The listing builds one solid part. Answer for the finished solid, in the listing's coordinates (mm). Give positions to 0.01 mm unless a question says otherwise; leave off trailing zeros. Order: outer loops, then holes, each group sorted by start corner. A loop starts at its lowest first (then second) coordinate and runs counter-clockwise, first axis right, second up. Notation, with made-up numbers: (37, 48) -> (87, 48) arc R28 cw to (87, 82) -> close; hole circle Ø5 at (78, -40). An arc over 180 degrees is marked (long way). One line per question, with ' | ' between items. Start each with the question number.
```python
from build123d import *

# Parameters (mm, degrees)
F0_R     = 0.5
F1_DEPTH = 3.175


# Not quite as in the source:
# - a length typed as a fraction of an inch, garbled in the dataset ("3 / 203.2 mm" for 3/8 in), is restored


with BuildPart() as f1:
    # F0 (on Top) → F1 (new body)
    with BuildSketch(Plane.XY):
        Polygon((-34.3393906951, 49.0726131633), (-37.3393906951, 49.0726131633), (-37.3393906951, 50.5726131633), (-38.8393906951, 50.5726131633), (-38.8393906951, 52.5726131633), (-37.3393906951, 52.5726131633), (-37.3393906951, 61.8976131633), (-41.3393906951, 61.8976131633), (-41.3393906951, 65.0726131633), (-47.3393906951, 65.0726131633), (-47.3393906951, 61.8976131633), (-47.3393906951, -21.1023868367), (-47.3393906951, -24.2773868367), (-41.3393906951, -24.2773868367), (-41.3393906951, -21.1023868367), (-37.3393906951, -21.1023868367), (-37.3393906951, -11.7773868367), (-38.8393906951, -11.7773868367), (-38.8393906951, -9.7773868367), (-37.3393906951, -9.7773868367), (-37.3393906951, -8.2773868367), (-34.3393906951, -8.2773868367), (-34.3393906951, -9.7773868367), (-32.8393906951, -9.7773868367), (-32.8393906951, -11.7773868367), (-34.3393906951, -11.7773868367), (-34.3393906951, -21.1023868367), (-30.3393906951, -21.1023868367), (-30.3393906951, -24.2773868367), (-24.3393906951, -24.2773868367), (-24.3393906951, -21.1023868367), (-24.3393906951, 61.8976131633), (-24.3393906951, 65.0726131633), (-30.3393906951, 65.0726131633), (-30.3393906951, 61.8976131633), (-34.3393906951, 61.8976131633), (-34.3393906951, 52.5726131633), (-32.8393906951, 52.5726131633), (-32.8393906951, 50.5726131633), (-34.3393906951, 50.5726131633), align=None)
        with Locations((-42.4286872149, -2.0273868367)):
            Circle(F0_R, mode=Mode.SUBTRACT)
        with Locations((-42.4286872149, 9.4726131633)):
            Circle(F0_R, mode=Mode.SUBTRACT)
        with Locations((-30.9286872149, -2.0273868367)):
            Circle(F0_R, mode=Mode.SUBTRACT)
        with Locations((-30.9286872149, 9.4726131633)):
            Circle(F0_R, mode=Mode.SUBTRACT)
    extrude(amount=F1_DEPTH)


solid = f1.part
```
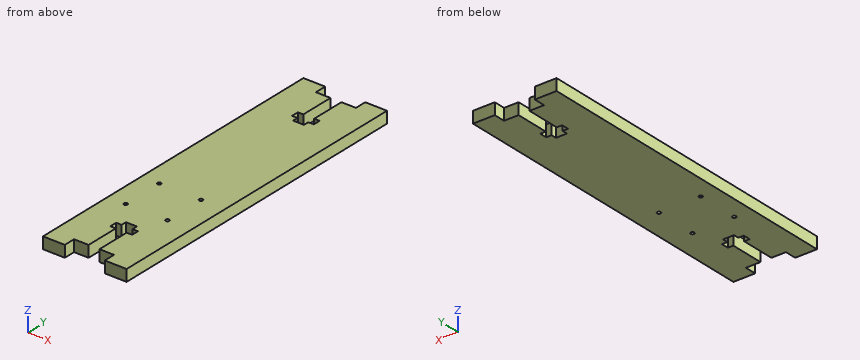
(1) Consider line 1 (Y direction, x = -42.5, z = 3.05); line 2 (Y direction, x = -38.75, z = 1.8); line 3 (X direction, y = -14, z = 2.75). Determine where each line is inside the solid, lowest interval first.
(2) The part is cut by section C-C on z = 2.2. State how many separate pieces and enclosed holes the cut face has, plus the area to 3 significant figures.
(3) The part is cut by section A-A on y = 57. Determine the outline of the cut face in (x, z) (3 decimals), plus the area to 3 significant figures.
(4) Given P1, Ø5, axis at x = -28, y = 30.5, coming from the -Z side; P2, Ø0.9, axis at x = -36.5, z = 1, coming from the +Y side; P3, Ø0.8, axis at x = -38, z = 2.5, coming from the +Y side; P4, Ø1.6, axis at x = -33.5, z = 1, coming from the -Y side, each flat-ended and moving along its own axis, determine where each tip first touches the part or whether it passes through.
(5) The part is cut by section B-B on x = -40. Determine the outline of the cut face in (y, z) (3 decimals), plus the area to 3 significant figures.
Result sheet:
1) line 1: y = -24.28 to -2.52, -1.53 to 8.98, 9.97 to 65.07 | line 2: y = -21.1 to -11.78, -9.78 to 50.57, 52.57 to 61.9 | line 3: x = -47.34 to -37.34, -34.34 to -24.34
2) separate pieces: 1 | enclosed holes: 4 | area: 1,890 mm^2
3) outline: (-47.339, 0) -> (-37.339, 0) -> (-37.339, 3.175) -> (-47.339, 3.175) -> close; (-34.339, 0) -> (-24.339, 0) -> (-24.339, 3.175) -> (-34.339, 3.175) -> close | area: 63.5 mm^2
4) P1: stops at z = 0 | P2: stops at y = 49.07 | P3: stops at y = 61.9 | P4: stops at y = -21.1
5) outline: (-21.102, 0) -> (61.898, 0) -> (61.898, 3.175) -> (-21.102, 3.175) -> close | area: 264 mm^2
